Print and shaded views of the part. All mm, measured from the part's lowest x, y and z. A direction names the side the tool comes from. Give positions to 0.01 mm unless a question says otherwise; leave off trailing zeros. Loops run counter-clockwise (first coordinate to the right, second up) from the corner with the lowest first, then second, coordinate; pieces in that order, holes last. Notation, with made-up numbers: M -22.75,68.25 L -0.75,68.25 A11 ccw -0.75,77.25 Z; hole C -27,-17.5 d4. An arc over 180 degrees is marked long. Answer in a Markdown table with one row per item.
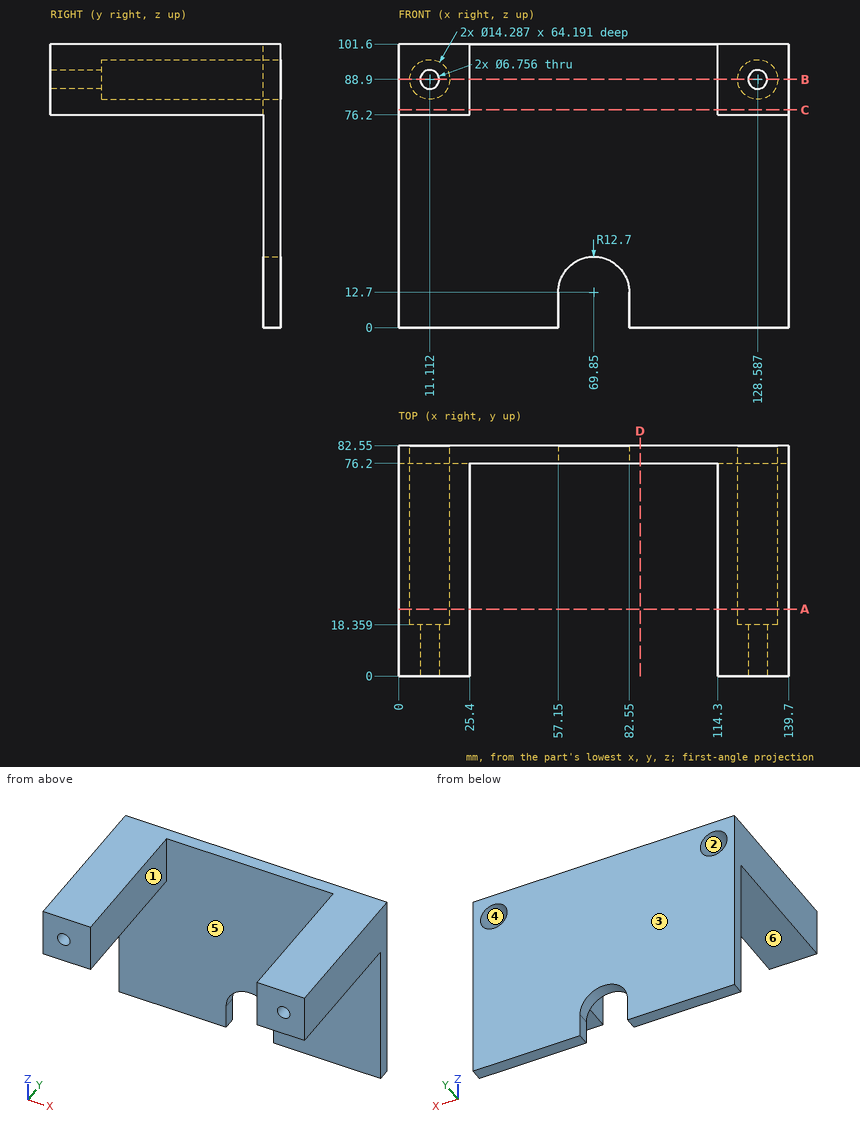
(1) Which spindle directions (+Z, -Z, +X, -X, +Y, -Y) get a long thin tool onto all of the face, cutting with end or side? Do the marked faces 1, 2 and 3. Say none if no direction does.
Established:
| item | result |
|---|---|
| face 1 | +Z, -Z, -Y |
| face 2 | +Y |
| face 3 | +Z, -Z, +X, -X, +Y |
(2) Saw through at A-A, the plane y = 24. Give the cut face in (x, z).
Established:
| item | result |
|---|---|
| outline | M 0,76.2 L 25.4,76.2 L 25.4,101.6 L 0,101.6 Z; M 114.3,76.2 L 139.7,76.2 L 139.7,101.6 L 114.3,101.6 Z; hole C 11.11,88.9 d14.29; hole C 128.59,88.9 d14.29 |
(3) Saw through at C-C, the plane z = 78. Give the cut face in (x, y), and give its area (3 significant figures).
Established:
| item | result |
|---|---|
| outline | M 0,0 L 25.4,0 L 25.4,76.2 L 114.3,76.2 L 114.3,0 L 139.7,0 L 139.7,82.55 L 0,82.55 Z |
| area | 4,760 mm2 |
(4) Wall check: L1, parallel to X at y = 47, z = 88.9; L2, parallel to X at y = 12.75, z = 88.9 (1 decimal); L3, parallel to X at y = 18, z = 79.5. Give the ranges that are in metal, low to high.
Established:
| item | result |
|---|---|
| L1 | x = 0 to 3.97, 18.26 to 25.4, 114.3 to 121.44, 135.73 to 139.7 |
| L2 | x = 0 to 7.7, 14.5 to 25.4, 114.3 to 125.2, 132 to 139.7 |
| L3 | x = 0 to 25.4, 114.3 to 139.7 |
(5) Mould opens along Z. For the marked faces 4, 5 and 6 say: pulls with the +Z half, pulls with the -Z half, needs draft (parallel to the pull), parting line crosses it, or undercut.
Established:
| item | result |
|---|---|
| face 4 | undercut |
| face 5 | needs draft |
| face 6 | pulls with the -Z half |
(6) Saw through at D-D, the plane x = 86.5. Give the cut face in (y, z), and give its area (3 significant figures).
Established:
| item | result |
|---|---|
| outline | M 76.2,0 L 82.55,0 L 82.55,101.6 L 76.2,101.6 Z |
| area | 645 mm2 |
(7) Flat gauge pins, fed straight in: P1, Ø13, axis at x = 11.11, z = 88.9, coming from the +Y side; P2, Ø12.5, axis at x = 127.5, y = 39, coming from the -Z side; P3, Ø6, axis at x = 111.5, y = 25, coming from the +Z side. Where does each tip first touch, or does it go through?
Established:
| item | result |
|---|---|
| P1 | stops at y = 18.36 |
| P2 | stops at z = 76.2 |
| P3 | stops at z = 101.6 |
(8) Saw through at B-B, the plane z = 88.9. Count the separate pieces of the cut face and the enclosed holes in it.
Established:
| item | result |
|---|---|
| separate pieces | 3 |
| enclosed holes | 0 |
